Design review of the part built by this model. Coordinates are the model's own, in mm. A direction names the side the tool comes from. Coordinates: 2 decimals unless noted, no trailing zeros. Write each loop counter-clockwise with the first axis right and the second up, starting at its lowest first coordinate (ties: lowest second). Pieces come first, ordered by that corner, then holes. Notation, with made-up numbers: (29.25, -28) -> (73.25, -28) arc R20 ccw to (73.25, -12) -> close; hole circle Ø2 at (4.25, -33). An arc over 180 degrees is marked (long way). Write item = value, one per line. Start each with the question number.
```python
from build123d import *

# Parameters (mm, degrees)
F0_R     = 27.5
F1_DEPTH = 28
F2_W     = 25
F2_H     = 6
F4_R     = 7
F5_DEPTH = 28.001


with BuildPart() as f1:
    # F0 (on Front) → F1 (new body)
    with BuildSketch(Plane.XZ):
        Circle(F0_R)
    extrude(amount=F1_DEPTH)

    # F2 (on Right) → F3 (revolve, cut)
    with BuildSketch(Plane.YZ):
        with Locations((-14, 24.5)):
            Rectangle(F2_W, F2_H)
    revolve(axis=Axis((0, 0, 0), (0, 1, 0)), mode=Mode.SUBTRACT)

    # F4 (on Front) → F5 (cut, through all)
    with BuildSketch(Plane.XZ):
        Circle(F4_R)
    extrude(amount=F5_DEPTH, mode=Mode.SUBTRACT)


solid = f1.part
```
(1) Take a section at B-B, the plane x = 0. State the section outline as (y, z) points.
(2) Take a section at D-D, the plane z = 18. State the section outline as (x, y) points, then the cut area to 3 significant figures.
(3) For faces 1 (the face through (21.317, -13.825, -2.799)), 2 (the face through (6.466, -13.804, -2.681)), list the 3-axis set-ups (+Z, -Z, +X, -X, +Y, -Y) from which the entire face can be reached by the end or side of a thin tool; tool diameter is ignored.
(4) For line 1 (X direction, y = -17, z = 0); line 2 (Y direction, x = 12.5, z = 19); line 3 (Z direction, x = 3, y = -17.5), list the stretches that pass through material, from the lowest coordinate up.
(5) Mouldability with a two-part tool opening along Y and no side actions: class faces 3 (the face through (25.403, -0.74, -10.533)), 4 (the face through (-14.13, -1.5, 16.42)), 5 (the face through (-14.13, -26.5, 16.42)), 6 (the face through (6, 0, -6)) as pulls with the +Y half, pulls with the -Y half, needs draft (parallel to the pull), parting line crosses it, or undercut.
(6) Take a section at C-C, the plane y = -14.5. State the section outline as (x, z) points.
(7) For pin 1 Ø1 at (x, y) = (-5, -23.5) entering from -Z; pin 2 Ø6 at (x, z) = (10, 7) entering from +Y; pin 3 Ø3 at (x, y) = (-2.5, -19) entering from +Z; pin 4 Ø2 at (y, z) = (-6, 16) entering from +X, all flat-tipped, find the tip position at first contact; note any pin that passes through.
(8) Take a section at A-A, the plane z = 0. State the section outline as (x, y) points.
Report:
q1.outline = (-28, -27.5) -> (-26.5, -27.5) -> (-26.5, -21.5) -> (-1.5, -21.5) -> (-1.5, -27.5) -> (0, -27.5) -> (0, -7) -> (-28, -7) -> close; (-28, 7) -> (0, 7) -> (0, 27.5) -> (-1.5, 27.5) -> (-1.5, 21.5) -> (-26.5, 21.5) -> (-26.5, 27.5) -> (-28, 27.5) -> close
q2.outline = (-20.79, -28) -> (20.79, -28) -> (20.79, -26.5) -> (11.76, -26.5) -> (11.76, -1.5) -> (20.79, -1.5) -> (20.79, 0) -> (-20.79, 0) -> (-20.79, -1.5) -> (-11.76, -1.5) -> (-11.76, -26.5) -> (-20.79, -26.5) -> close
q2.area = 713 mm2
q3.face_1 = none
q3.face_2 = +Y, -Y
q4.line_1 = -21.5 to -7, 7 to 21.5
q4.line_2 = -28 to -26.5, -1.5 to 0
q4.line_3 = -21.29 to -6.32, 6.32 to 21.29
q5.face_3 = needs draft
q5.face_4 = undercut
q5.face_5 = undercut
q5.face_6 = pulls with the +Y half
q6.outline = circle Ø43 at (0, 0); hole circle Ø14 at (0, 0)
q7.pin_1 = -21.02
q7.pin_2 = 0
q7.pin_3 = 21.48
q7.pin_4 = 15.4
q8.outline = (-27.5, -28) -> (-7, -28) -> (-7, 0) -> (-27.5, 0) -> (-27.5, -1.5) -> (-21.5, -1.5) -> (-21.5, -26.5) -> (-27.5, -26.5) -> close; (7, -28) -> (27.5, -28) -> (27.5, -26.5) -> (21.5, -26.5) -> (21.5, -1.5) -> (27.5, -1.5) -> (27.5, 0) -> (7, 0) -> close
